from build123d import *

# Parameters (mm, degrees)
F0_R     = 10.16
F1_DEPTH = 25.4
F2_W     = 25.4
F2_H     = 12.7
F3_DEPTH = 50.8
F4_W     = 12.7
F4_H     = 12.7
F5_DEPTH = 25.4
F6_SIZE  = 1.27


with BuildPart() as f1:
    # F0 (on Front) → F1 (new body)
    with BuildSketch(Plane.XZ):
        with BuildLine():
            Line((-19.05, 12.7), (-19.05, -31.75))
            Line((-19.05, -31.75), (19.05, -31.75))
            Line((19.05, -31.75), (19.05, 12.7))
            ThreePointArc((19.05, 12.7), (13.4703841797, 26.1703841835), (-5.4e-09, 31.75))
            ThreePointArc((-5.4e-09, 31.75), (-13.4703841835, 26.1703841797), (-19.05, 12.7))
        make_face()
        with Locations((0, 12.7)):
            Circle(F0_R, mode=Mode.SUBTRACT)
    extrude(amount=F1_DEPTH)

    # F2 (on face) → F3 (join)
    with BuildSketch(Plane.XZ.offset(25.4)):
        with Locations((-6.35, -25.4)):
            Rectangle(F2_W, F2_H)
    extrude(amount=F3_DEPTH)

    # F4 (on face) → F5 (join)
    with BuildSketch(Plane.XZ.offset(25.4)):
        with Locations((12.7, -25.4)):
            Rectangle(F4_W, F4_H)
    extrude(amount=F5_DEPTH)

    # F6
    f6_edges = [f1.edges().sort_by_distance(p)[0] for p in [
        (-19.05, -50.8, -19.05),
        (-6.35, -76.2, -19.05),
        (6.35, -63.5, -19.05),
        (12.7, -50.8, -19.05),
        (19.05, -38.1, -19.05),
    ]]
    chamfer(f6_edges, length=F6_SIZE)


solid = f1.part
Verification items for the finished model (mm, model axes). A direction names the side the tool comes from. Coordinates: 2 decimals unless noted, no trailing zeros. Order: outer loops, then holes, each group sorted by start corner. A loop starts at its lowest first (then second) coordinate and runs counter-clockwise, first axis right, second up. Notation, with made-up numbers: M 50.5,22.25 L 103.5,22.25 A26 ccw 103.5,57.25 Z; hole C 8,10.5 d10. An arc over 180 degrees is marked long. Write each question's results on one line, items separated by ' | '.
1) Scan lines: line 1 along Z through (x, y) = (0, -10.5); line 2 along Z through (x, y) = (-2, -35); line 3 along Y through (x, z) = (13, 24.5). Record each from-to range of solid material in increasing order. Write a range as [from, to].
Solved:
line 1: z = [-31.75, 2.54], [22.86, 31.75] | line 2: z = [-31.75, -19.05] | line 3: y = [-25.4, 0]
2) Section check A-A on x = -3. Record the cut outline in (y, z).
Solved:
outline: M -76.2,-31.75 L 0,-31.75 L 0,2.99 L -25.4,2.99 L -25.4,-19.05 L -74.93,-19.05 L -76.2,-20.32 Z; M -25.4,22.41 L 0,22.41 L 0,31.51 L -25.4,31.51 Z
3) Section check D-D on x = 2. Record the cut outline in (y, z), plus the area to 3 significant figures.
Solved:
outline: M -76.2,-31.75 L 0,-31.75 L 0,2.74 L -25.4,2.74 L -25.4,-19.05 L -74.93,-19.05 L -76.2,-20.32 Z; M -25.4,22.66 L 0,22.66 L 0,31.64 L -25.4,31.64 Z | area: 1,750 mm²
4) Release check for a two-part mould opening along X. For faces 1 (the face through (-19.05, -21, -15)), 2 (the face through (19.05, -19, -15)), 3 (the face through (-2.2, -12.52, 2.78)), 4 (the face through (0, 0, -7)) record: pulls with the +X half, pulls with the -X half, needs draft (parallel to the pull), parting line crosses it, or undercut.
Solved:
face 1: pulls with the -X half | face 2: pulls with the +X half | face 3: undercut | face 4: needs draft
5) Section check C-C on y = -39. Record the cut outline in (x, z).
Solved:
outline: M -19.05,-31.75 L 19.05,-31.75 L 19.05,-20.32 L 17.78,-19.05 L -17.78,-19.05 L -19.05,-20.32 Z
6) Access from +Z, -Z, +X, -X, +Y, -Y to the whole of each face (thin tool, end or side, straight path). Record for faces 5 (the face through (6.35, -63, -26)), 6 (the face through (-4, -50, -19.05)), 7 (the face through (-7, -76.2, -26)).
Solved:
face 5: +Z, -Z, +X, -Y | face 6: +Z, +X, -X, -Y | face 7: +Z, -Z, +X, -X, -Y
7) Gauge pin test, flat ends, axial feed: pin 1 Ø1.5 at (x, y) = (-14, -46.5) entering from +Z; pin 2 Ø5.5 at (x, z) = (15.5, -24) entering from -Y; pin 3 Ø3.5 at (y, z) = (-64, -26) entering from +X. Record the tip position at first contact, or that the pin passes through.
Solved:
pin 1: stops at z = -19.05 | pin 2: stops at y = -50.8 | pin 3: stops at x = 6.35
8) Section check B-B on z = 5.5. Record the cut outline in (x, y).
Solved:
outline: M -19.05,-25.4 L -7.17,-25.4 L -7.17,0 L -19.05,0 Z; M 7.17,-25.4 L 19.05,-25.4 L 19.05,0 L 7.17,0 Z
